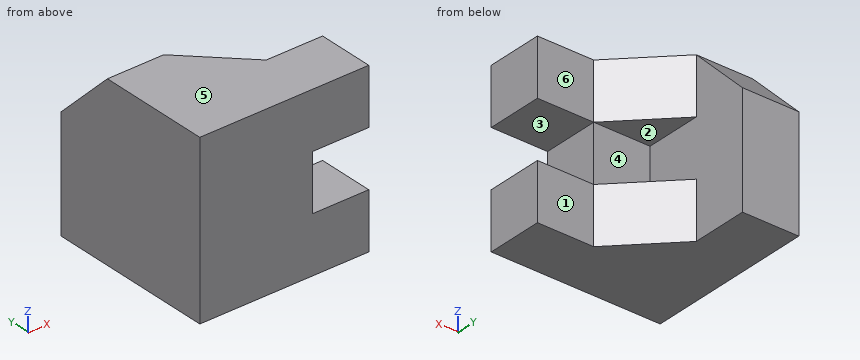
```python
from build123d import *

# Parameters (mm, degrees)
SALIENTE_EXTRUIR1_DEPTH = 60
CORTAR_EXTRUIR1_DEPTH   = 20
CROQUIS6_W              = 20
CROQUIS6_H              = 20
CORTAR_EXTRUIR3_DEPTH   = 10


with BuildPart() as part:
    # Croquis3 → Saliente-Extruir1 (new body)
    with BuildSketch(Plane.XY):
        Polygon((0, 0), (60, 0), (60, 20), (40, 20), (20, 40), (20, 60), (0, 60), align=None)
    extrude(amount=-SALIENTE_EXTRUIR1_DEPTH)

    # Croquis4 → Cortar-Extruir1 (cut)
    with BuildSketch(Plane(origin=(20, 0, 0), x_dir=(0, 0, -1), z_dir=(1, 0, 0))):
        Polygon((0, 40), (20, 60), (0, 60), align=None)
    extrude(amount=-CORTAR_EXTRUIR1_DEPTH, mode=Mode.SUBTRACT)

    # Croquis6 → Cortar-Extruir3 (cut, symmetric)
    with BuildSketch(Plane.XY.offset(-30)):
        Polygon((20, 40), (20, 20), (40, 20), align=None)
        with Locations((50, 10)):
            Rectangle(CROQUIS6_W, CROQUIS6_H)
    extrude(amount=CORTAR_EXTRUIR3_DEPTH, both=True, mode=Mode.SUBTRACT)


solid = part.part
```
Geometry check sheet. Reference: the model listing, model coordinates, mm. Face numbers are marked on the shaded views. A direction names the side the tool comes from. Coordinates: 2 decimals unless noted, no trailing zeros. Loops run counter-clockwise (first coordinate to the right, second up) from the corner with the lowest first, then second, coordinate; pieces in that order, holes last. Notation, with made-up numbers: (89.5, 3.5) -> (118.5, 3.5) arc R24 cw to (118.5, 30.5) -> close; hole circle Ø1 at (21.5, 5). An arc over 180 degrees is marked (long way). Put each result on its own line as item: value.
1) Cross-section at B-B on x = 27.5. Record the boundary of the cut face in (y, z).
Result set:
outline: (0, -60) -> (32.5, -60) -> (32.5, -40) -> (20, -40) -> (20, -20) -> (32.5, -20) -> (32.5, 0) -> (0, 0) -> close
2) Gauge pin test, flat ends, axial feed: pin 1 Ø8 at (y, z) = (30, -19.5) entering from +X; pin 2 Ø5 at (y, z) = (27, -28) entering from -X; pin 3 Ø10 at (x, z) = (51.5, -46.5) entering from +Y; pin 4 Ø4 at (y, z) = (48, -12.5) entering from +X. Record the tip position at first contact, or that the pin passes through.
Result set:
pin 1: stops at x = 34
pin 2: stops at x = 0
pin 3: stops at y = 20
pin 4: stops at x = 20
3) Thickness scan on line 1 (Z direction, x = 57.5, y = 6); line 2 (X direction, y = 53.5, z = -39). Record the ranges inside material, lowest first.
Result set:
line 1: z = -60 to -40, -20 to 0
line 2: x = 0 to 20
4) Cross-section at D-D on z = -27.5. Record the boundary of the cut face in (x, y), plus the area to 3 significant figures.
Result set:
outline: (0, 0) -> (40, 0) -> (40, 20) -> (20, 20) -> (20, 60) -> (0, 60) -> close
area: 1,600 mm^2
5) Cross-section at A-A on z = -54. Record the boundary of the cut face in (x, y), plus the area to 3 significant figures.
Result set:
outline: (0, 0) -> (60, 0) -> (60, 20) -> (40, 20) -> (20, 40) -> (20, 60) -> (0, 60) -> close
area: 2,200 mm^2
6) Tool access check on the marked faces 1, 2 and 3. Record the directions out of +Z, -Z, +X, -X, +Y, -Y that give a thin tool (end or side, any length) a straight path to the whole face; none if there is none.
Result set:
face 1: +Z, -Z, +X, +Y
face 2: +X, +Y
face 3: +X, +Y, -Y
7) Release check for a two-part mould opening along Z. For the marked faces 4, 5 and 6 record: released by +Z, released by -Z, zero draft, split by the parting line, or undercut.
Result set:
face 4: undercut
face 5: released by +Z
face 6: zero draft
8) Cross-section at C-C on y = 36. Record the boundary of the cut face in (x, z), plus the area to 3 significant figures.
Result set:
outline: (0, -60) -> (24, -60) -> (24, -40) -> (20, -40) -> (20, -20) -> (24, -20) -> (24, 0) -> (0, 0) -> close
area: 1,360 mm^2
